The drawing under review shows one solid part. Ordinate dimensions are in mm from its lowest x, y, z. A direction names the side the tool comes from. Coordinates: 2 decimals unless noted, no trailing zeros. Order: outer loops, then holes, each group sorted by start corner. A loop starts at its lowest first (then second) coordinate and runs counter-clockwise, first axis right, second up. Notation, with made-up numbers: (86, 57.5) -> (117, 57.5) arc R5 ccw to (117, 66.5) -> close; hole circle Ø3 at (15.5, -30.5). An arc over 180 degrees is marked (long way). Use a Markdown table: item, result. Add a question column.
Q1. Wall thickness on probe 1 along X at (y, z) = (64, 8.5); probe 2 along Y at (x, z) = (46.5, 14); probe 3 along X at (y, z) = (54.5, 1.5): over which ranges is each line inside the solid? List them lowest first.
Q2. Add section A-A (y = 51). State the section outline as (x, z) points, then the cut area to 3 significant figures.
Q3. Add section D-D (x = 47). State the section outline as (y, z) points, then the cut area to 3 significant figures.
Q4. The part is to be moulded in two halves that separate along Y. For the marked faces 1, 2, 3 and 4, say which applies: pulls with the +Y half, pulls with the -Y half, needs draft (parallel to the pull), parting line crosses it, or undercut.
Q5. Add section C-C (x = 38.5). State the section outline as (y, z) points, then the cut area to 3 significant figures.
Q6. Insertion check: pin 1 (12 mm diameter, centred on x = 39.5, y = 29.5, fed in from -Z); pin 2 (0.5 mm diameter, centred on x = 50.5, z = 1.5, fed in from +Y); pin 3 (10 mm diameter, centred on x = 25.5, z = 9, fed in from -Y). Each pin has a flat end and moves straight along its axis. Give the tip position at first contact, or say it passes through.
Q7. Add section B-B (z = 6). State the section outline as (x, y) points.
Q8. Machinability: for the marked faces 5 and 6, which of the approach directions +Z, -Z, +X, -X, +Y, -Y give a long, thin tool a straight path to every point of the face, cutting with its end or side? Answer none if there is none.
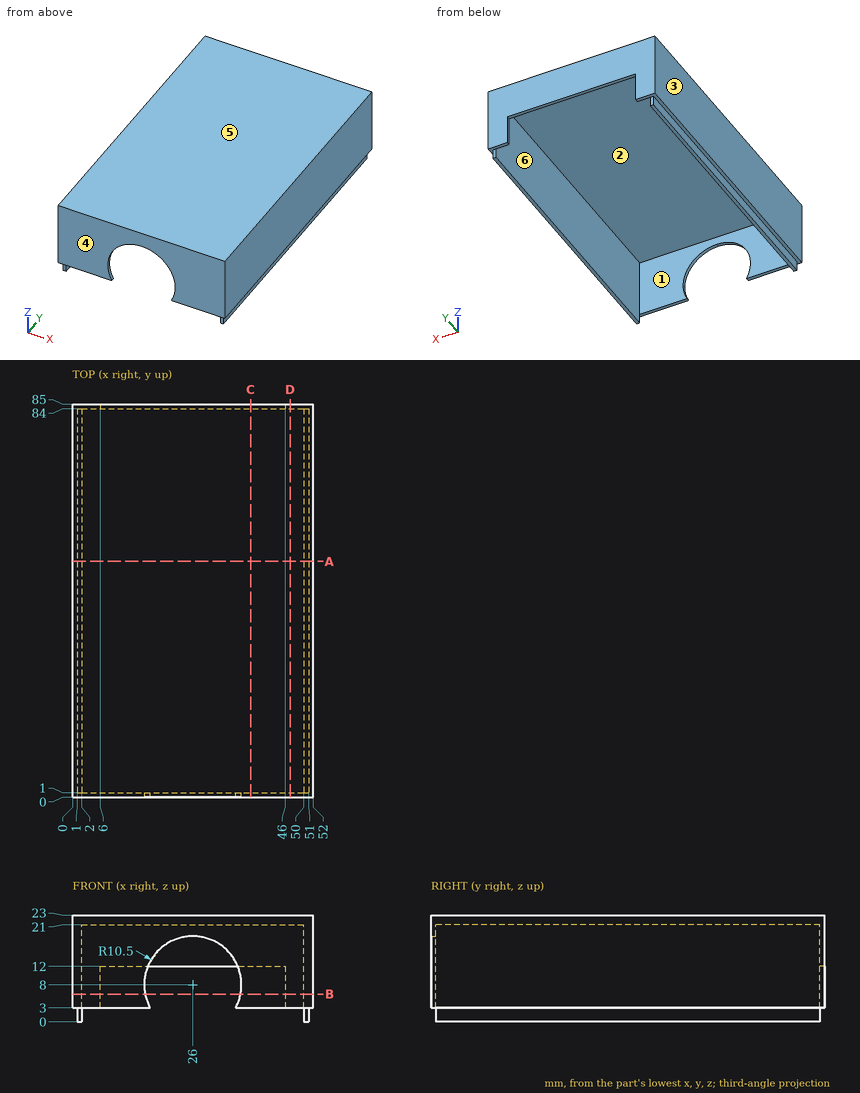
Established:
| question | item | result |
|---|---|---|
| 1 | probe 1 | 0 to 2, 50 to 52 |
| 1 | probe 2 | 0 to 1, 84 to 85 |
| 1 | probe 3 | 1 to 2, 50 to 51 |
| 2 | outline | (0, 3) -> (1, 3) -> (1, 0) -> (2, 0) -> (2, 21) -> (50, 21) -> (50, 0) -> (51, 0) -> (51, 3) -> (52, 3) -> (52, 23) -> (0, 23) -> close |
| 2 | area | 182 mm^2 |
| 3 | outline | (0, 3) -> (1, 3) -> (1, 21) -> (84, 21) -> (84, 3) -> (85, 3) -> (85, 23) -> (0, 23) -> close |
| 3 | area | 206 mm^2 |
| 4 | face 1 | undercut |
| 4 | face 2 | undercut |
| 4 | face 3 | needs draft |
| 4 | face 4 | pulls with the -Y half |
| 5 | outline | (0, 3) -> (1, 3) -> (1, 21) -> (84, 21) -> (84, 12) -> (85, 12) -> (85, 23) -> (0, 23) -> close |
| 5 | area | 197 mm^2 |
| 6 | pin 1 | z = 21 |
| 6 | pin 2 | y = 84 |
| 6 | pin 3 | y = 84 |
| 7 | outline | (0, 0) -> (15.69, 0) -> (15.69, 1) -> (2, 1) -> (2, 84) -> (6, 84) -> (6, 85) -> (0, 85) -> close; (36.31, 0) -> (52, 0) -> (52, 85) -> (46, 85) -> (46, 84) -> (50, 84) -> (50, 1) -> (36.31, 1) -> close |
| 8 | face 5 | +Z, +X, -X, +Y, -Y |
| 8 | face 6 | -Z |
